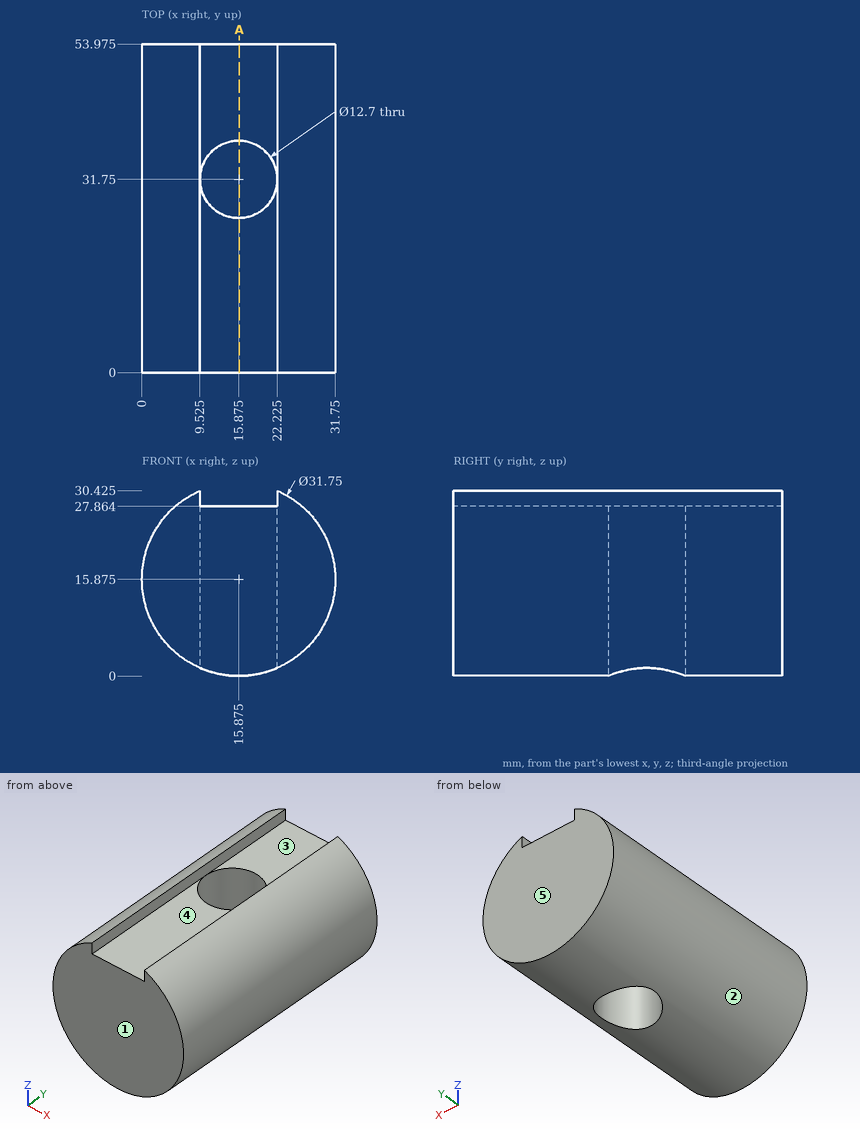
Answer from the drawing. Dimensions are ordinates in mm from the lowest x, y and z of the part. A direction names the side the tool comes from. Coordinates: 2 decimals unless noted, no trailing zeros. Loops run counter-clockwise (first coordinate to the right, second up) from the corner with the lowest first, then second, coordinate; pieces in that order, holes last.
Q1. Each of these flat-tipped pins is pushed along its axis until it touches: pin 1 Ø14 at (x, y) = (17.5, 13.5) entering from +Z (1 decimal); pin 2 Ø0.8 at (y, z) = (39, 29) entering from -X (1 decimal); pin 3 Ø3 at (x, y) = (22.5, 41.5) entering from -Z. Where does it stop, or does it pass through?
Q2. Which of the six approach directions +Z, -Z, +X, -X, +Y, -Y give full straight-line access (tool end or side, diameter ignored) to the marked faces 4 and 5?
Q3. The part is cut by section A-A on x = 16. Write down the section's boundary in (y, z) (1 decimal).
Q4. The mould has two halves that part along X. Classify the marked faces 1, 2 and 3: +X half, -X half, draft (parallel to the pull), parting line (faces both ways), or undercut.
Q5. Consider probe 1 along X at (y, z) = (31.5, 16); probe 2 along X at (y, z) = (31, 7); probe 3 along Y at (x, z) = (21.5, 11.5) (1 decimal). Determine where each line is inside the solid, lowest interval first.
Results below:
1. pin 1: stops at z = 30.4
1. pin 2: stops at x = 6.4
1. pin 3: stops at z = 0.85
2. face 4: +Z, +Y, -Y
2. face 5: +Z, -Z, +X, -X, +Y
3. outline: (0, 0) - (25.4, 0) - (25.4, 27.9) - (0, 27.9) - close; (38.1, 0) - (54, 0) - (54, 27.9) - (38.1, 27.9) - close
4. face 1: draft
4. face 2: parting line
4. face 3: undercut
5. probe 1: x = 0 to 9.53, 22.22 to 31.75
5. probe 2: x = 2.71 to 9.57, 22.18 to 29.04
5. probe 3: y = 0 to 28.8, 34.7 to 54
